from build123d import *

# Parameters (mm, degrees)
CROQUIS1_R              = 1.75
SALIENTE_EXTRUIR1_DEPTH = 4


with BuildPart() as part:
    # Croquis1 → Saliente-Extruir1 (new body)
    with BuildSketch(Plane(origin=(0, 0, 0), x_dir=(1, 0, 0), z_dir=(0, 1, 0))):
        Polygon((-26, -12.5), (-50, -12.5), (-50, -37.5), (50, -37.5), (50, -12.5), (26, -12.5), (26, 37.5), (-26, 37.5), align=None)
        with Locations(Location((-38, -25.816065761, 0), (0, 0, 270))):
            Circle(CROQUIS1_R, mode=Mode.SUBTRACT)
        with Locations(Location((-38, -18.479827089, 0), (0, 0, 270))):
            Circle(CROQUIS1_R, mode=Mode.SUBTRACT)
        with Locations(Location((0, -9.329285485, 0), (0, 0, 270))):
            Circle(CROQUIS1_R, mode=Mode.SUBTRACT)
        with Locations(Location((0, -1.504051409, 0), (0, 0, 270))):
            Circle(CROQUIS1_R, mode=Mode.SUBTRACT)
        with Locations(Location((38, -25.816065761, 0), (0, 0, 270))):
            Circle(CROQUIS1_R, mode=Mode.SUBTRACT)
        with Locations(Location((38, -18.479827089, 0), (0, 0, 270))):
            Circle(CROQUIS1_R, mode=Mode.SUBTRACT)
        with Locations(Location((0, 32.46376687, 0), (0, 0, 270))):
            Circle(CROQUIS1_R, mode=Mode.SUBTRACT)
    extrude(amount=SALIENTE_EXTRUIR1_DEPTH)


solid = part.part
Read the model definition and answer for the solid it produces. Units are mm, in the model's axes. A direction names the side the tool comes from. Give positions to 0.01 mm unless a question says otherwise; leave off trailing zeros. Loops run counter-clockwise (first coordinate to the right, second up) from the corner with the lowest first, then second, coordinate; pieces in that order, holes last. Notation, with made-up numbers: (19.25, 19.25) -> (64.25, 19.25) arc R11 ccw to (64.25, 33.25) -> close; hole circle Ø2 at (-21.75, 57.25). An arc over 180 degrees is marked (long way). Answer as CSV lines item,"result".
Item 1: For faces 1 (the face through (38, 2, 12.5)), 2 (the face through (-39.065, 1.972, 17.091)), determine the directions among +Z, -Z, +X, -X, +Y, -Y from which every point of the face is accessible in a straight line to the end or side of a thin tool.
Returned:
face 1,"-Z, +X, +Y, -Y"
face 2,"+Y, -Y"
Item 2: Consider line 1 (X direction, y = 1.85, z = -4.5); line 2 (X direction, y = 2.9, z = -31.5); line 3 (Z direction, x = -45.5, y = 3.85). Determine where each line is inside the solid, lowest interval first. Write a range as [from, to].
Returned:
line 1,"x = [-26, 26]"
line 2,"x = [-26, -1.46], [1.46, 26]"
line 3,"z = [12.5, 37.5]"
Item 3: Each of these flat-tipped pins is pushed along its axis until it touches: pin 1 (2 mm diameter, centred on y = 1, z = -11.5, fed in from +X); pin 2 (2 mm diameter, centred on y = 2.5, z = -1.5, fed in from -X); pin 3 (2 mm diameter, centred on x = 35, y = 2.5, fed in from -Z); pin 4 (4 mm diameter, centred on x = 0, z = -32.46, fed in from -Y). Where does it stop, or does it pass through?
Returned:
pin 1,"stops at x = 26"
pin 2,"stops at x = -26"
pin 3,"stops at z = 12.5"
pin 4,"stops at y = 0"
Item 4: Find section C-C on x = -38. Give the vertices of the cut face in (y, z).
Returned:
outline,"(0, 12.5) -> (4, 12.5) -> (4, 16.73) -> (0, 16.73) -> close; (0, 20.23) -> (4, 20.23) -> (4, 24.07) -> (0, 24.07) -> close; (0, 27.57) -> (4, 27.57) -> (4, 37.5) -> (0, 37.5) -> close"
Item 5: Find section B-B on y = 1.75. Give the vertices of the cut face in (x, z).
Returned:
outline,"(-50, 12.5) -> (-26, 12.5) -> (-26, -37.5) -> (26, -37.5) -> (26, 12.5) -> (50, 12.5) -> (50, 37.5) -> (-50, 37.5) -> close; hole circle Ø3.5 at (-38, 18.48); hole circle Ø3.5 at (-38, 25.82); hole circle Ø3.5 at (0, -32.46); hole circle Ø3.5 at (0, 1.5); hole circle Ø3.5 at (0, 9.33); hole circle Ø3.5 at (38, 18.48); hole circle Ø3.5 at (38, 25.82)"
Item 6: Find section A-A on x = 0. Give the vertices of the cut face in (y, z), plus the area to 3 significant figures.
Returned:
outline,"(0, -37.5) -> (4, -37.5) -> (4, -34.21) -> (0, -34.21) -> close; (0, -30.71) -> (4, -30.71) -> (4, -0.25) -> (0, -0.25) -> close; (0, 3.25) -> (4, 3.25) -> (4, 7.58) -> (0, 7.58) -> close; (0, 11.08) -> (4, 11.08) -> (4, 37.5) -> (0, 37.5) -> close"
area,"258 mm²"
Item 7: Find section D-D on z = 18. Give the vertices of the cut face in (x, y).
Returned:
outline,"(-50, 0) -> (-39.68, 0) -> (-39.68, 4) -> (-50, 4) -> close; (-36.32, 0) -> (36.32, 0) -> (36.32, 4) -> (-36.32, 4) -> close; (39.68, 0) -> (50, 0) -> (50, 4) -> (39.68, 4) -> close"
Item 8: Determine the mould class of faces 3 (the face through (-38, 2, 12.5)), 4 (the face through (37.33, 1.972, 27.433)), 5 (the face through (-26, 2, -13)) for opening direction Z: +Z half, -Z half, draft (parallel to the pull), parting line (faces both ways), or undercut.
Returned:
face 3,"-Z half"
face 4,"undercut"
face 5,"draft"
